Autodesk Inventor part; units mm, degrees
ref_plane "YZ Plane" through (0, 0, 0) normal (1, 0, 0) x (0, 1, 0)
ref_plane "XZ Plane" through (0, 0, 0) normal (0, 1, 0) x (-1, 0, 0)
ref_plane "XY Plane" through (0, 0, 0) normal (0, 0, 1) x (1, 0, 0)
sketch "Sketch1" plane through (0, 0, 0) normal (0, 0, 1) x (1, 0, 0)
  line L0 (120, 0) -> (120, -100)
  line L1 (120, 0) -> (120, 100)
  line L2 (-60, 103.923) -> (26.6025, 153.923)
  line L3 (-60, 103.923) -> (-146.6025, 53.923)
  line L4 (-60, -103.923) -> (-146.6025, -53.923)
  line L5 (-60, -103.923) -> (26.6025, -153.923)
  line L6 (26.6025, 153.923) -> (120, 100)
  line L7 (120, -100) -> (26.6025, -153.923)
  line L8 (-146.6025, -53.923) -> (-146.6025, 53.923)
  circle A0 centre (0, 0) radius 10
  dimension "d5" = 360
extrude "Extrusion1" add sketch "Sketch1" along normal blind 8
sketch "Sketch2" plane through (0, 0, 8) normal (0, 0, 1) x (1, 0, 0)
  circle A0 centre (84.2544, -15) radius 2.5
  line L0 (120, -100) -> (120, 100)
  circle A1 centre (84.2544, -35) radius 2.5
  circle A2 centre (54.2544, -15) radius 2.5
  circle A3 centre (54.2544, -35) radius 2.5
  circle A4 centre (-14.1368, 54.4857) radius 2.5
  circle A5 centre (-29.1368, 80.4664) radius 2.5
  circle A6 centre (-11.8163, 90.4664) radius 2.5
  circle A7 centre (3.1837, 64.4857) radius 2.5
  circle A8 centre (-40.1176, -39.4857) radius 2.5
  circle A9 centre (-55.1176, -65.4664) radius 2.5
  circle A10 centre (-72.4381, -55.4664) radius 2.5
  circle A11 centre (-57.4381, -29.4857) radius 2.5
  point P0 (0, 0)
  point P1 (120, 0)
  dimension "d11" = 5
  dimension "d12" = 15
  dimension "d13" = 5
  dimension "d14" = 20
  dimension "d15" = 5
  dimension "d16" = 5
  dimension "d17" = 20
  dimension "d18" = 30
  dimension "d21" = 360
extrude "Extrusion2" cut sketch "Sketch2" against normal blind 8
sketch "Sketch3" plane through (0, 0, 8) normal (0, 0, 1) x (1, 0, 0)
  circle A0 centre (-136.6025, 35) radius 2.5
  circle A1 centre (-136.6025, 0) radius 2.5
  circle A2 centre (-136.6025, -35) radius 2.5
  line L0 (-146.6025, 53.923) -> (-146.6025, -53.923)
  circle A3 centre (37.9904, -135.8013) radius 2.5
  circle A4 centre (68.3013, -118.3013) radius 2.5
  circle A5 centre (98.6122, -100.8013) radius 2.5
  circle A6 centre (98.6122, 100.8013) radius 2.5
  circle A7 centre (68.3013, 118.3013) radius 2.5
  circle A8 centre (37.9904, 135.8013) radius 2.5
  point P0 (0, 0)
  point P1 (-146.6025, 0)
  point P2 (-146.6025, 0)
  dimension "d25" = 5
  dimension "d26" = 5
  dimension "d27" = 5
  dimension "d28" = 35
  dimension "d29" = 35
  dimension "d30" = 0
  dimension "d33" = 360
  dimension "d82" = 10
  dimension "d83" = 10
extrude "Extrusion3" cut sketch "Sketch3" against normal blind 8
sketch "Sketch5" plane through (0, 0, 8) normal (0, 0, 1) x (1, 0, 0)
  circle A0 centre (18.3712, 0) radius 2.5
  circle A1 centre (9.1856, 15.9099) radius 2.5
  circle A2 centre (-9.1856, 15.9099) radius 2.5
  circle A3 centre (-18.3712, 0) radius 2.5
  circle A4 centre (-9.1856, -15.9099) radius 2.5
  circle A5 centre (9.1856, -15.9099) radius 2.5
  point P0 (0, 0)
  dimension "d51" = 5
  dimension "d54" = 360
extrude "Extrusion5" cut sketch "Sketch5" against normal blind 8
sketch "Sketch6" plane through (0, 0, 8) normal (0, 0, 1) x (1, 0, 0)
  circle A0 centre (53.9473, 40) radius 2.5
  circle A1 centre (53.9473, 20) radius 2.5
  line L0 (120, -100) -> (120, 100)
  circle A2 centre (-70.3891, 40) radius 2.5
  circle A3 centre (-70.3891, 20) radius 2.5
  point P0 (0, 0)
  point P1 (120, 0)
  dimension "d58" = 5
  dimension "d59" = 5
  dimension "d60" = 20
  dimension "d61" = 20
  dimension "d62" = 5
  dimension "d63" = 5
  dimension "d64" = 20
extrude "Extrusion6" cut sketch "Sketch6" against normal blind 8
sketch "Sketch7" plane through (0, 0, 8) normal (0, 0, 1) x (1, 0, 0)
  circle A0 centre (110, 0) radius 2.5
  circle A1 centre (110, 50) radius 2.5
  circle A2 centre (110, -50) radius 2.5
  line L0 (120, -100) -> (120, 100)
  circle A3 centre (-98.3013, 70.2628) radius 2.5
  circle A4 centre (-55, 95.2628) radius 2.5
  circle A5 centre (-11.6987, 120.2628) radius 2.5
  circle A6 centre (-11.6987, -120.2628) radius 2.5
  circle A7 centre (-55, -95.2628) radius 2.5
  circle A8 centre (-98.3013, -70.2628) radius 2.5
  point P0 (0, 0)
  point P1 (120, 0)
  point P2 (120, 0)
  point P3 (120, 0)
  dimension "d68" = 5
  dimension "d69" = 5
  dimension "d70" = 5
  dimension "d71" = 50
  dimension "d72" = 50
  dimension "d75" = 360
  dimension "d77" = 10
  dimension "d78" = 10
  dimension "d79" = 10
extrude "Extrusion7" cut sketch "Sketch7" against normal blind 8
equation "\"BendRadius\" = Thickness"
equation "\"BendReliefWidth\" = Thickness"
equation "\"BendReliefDepth\" = 0.5 * Thickness"
equation "\"CornerReliefSize\" = 4 * Thickness"
equation "\"MinimumRemnant\" = 2 * Thickness"
equation "\"TransitionRadius\" = BendRadius"
equation "\"JacobiRadiusSize\" = BendRadius"
equation "\"GapSize\" = Thickness"
properties part number "đế trên"
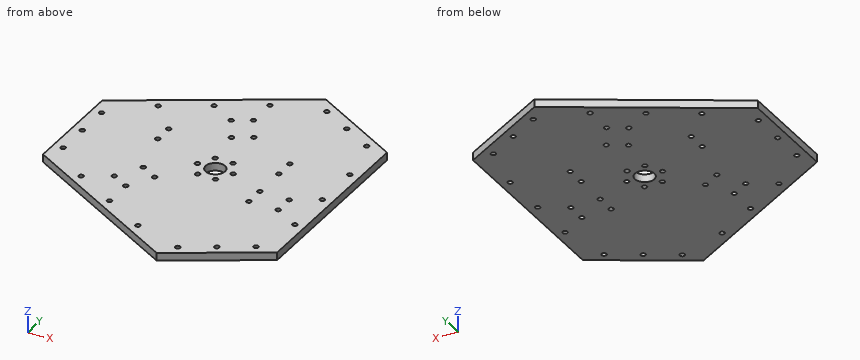
For this review, take the finished solid that the model builds, in its own axes (mm). Coordinates: 2 decimals unless noted, no trailing zeros. Write each loop counter-clockwise with the first axis right and the second up, starting at its lowest first coordinate (ties: lowest second). Pieces come first, ordered by that corner, then holes.
(1) Add section B-B on y = -81.5. Give the boundary of the cut face in (x, z).
(2) Wall thickness on probe 1 along Y at (x, z) = (109.5, 4.5); probe 2 along X at (y, z) = (17, 4.25); probe 3 along Y at (x, z) = (-57, 4): over which ranges is each line inside the solid? List them lowest first.
(3) Add section A-A on z = 4.5. Count the separate pieces of the cut face and the enclosed holes in it, then the cut area to 3 significant figures.
(4) Add section C-C on x = 61.5. Give the boundary of the cut face in (y, z), then the cut area to 3 significant figures.
(5) For pin 1 Ø2 at (x, z) = (-107, 1) entering from +Y; pin 2 Ø4 at (y, z) = (-109.5, 2) entering from -X, all flat-tipped, find the tip position at first contact; note any pin that passes through.
Answer sheet:
1. outline: (-98.84, 0) - (120, 0) - (120, 8) - (-98.84, 8) - close
2. probe 1: y = -106.06 to -52.45, -47.55 to -2.45, 2.45 to 47.55, 52.45 to 106.06
2. probe 2: x = -146.6 to -11.44, -6.94 to 6.94, 11.44 to 120
2. probe 3: y = -105.66 to -96.76, -93.76 to -67.11, -63.82 to -31.95, -27.02 to 93.76, 96.76 to 105.66
3. separate pieces: 1
3. enclosed holes: 41
3. area: 58,600 mm2
4. outline: (-133.77, 0) - (133.77, 0) - (133.77, 8) - (-133.77, 8) - close
4. area: 2,140 mm2
5. pin 1: stops at y = 77.36
5. pin 2: stops at x = -53.8
